```python
from build123d import *

# Parameters (mm, degrees)
SKIZZE1_W                       = 22
SKIZZE1_H                       = 72.8
AUFSATZ_LINEAR_AUSTRAGEN1_DEPTH = 2
SKIZZE2_R                       = 3
SCHNITT_LINEAR_AUSTRAGEN1_DEPTH = 2
SKIZZE3_W                       = 65.5
SKIZZE3_H                       = 21
AUFSATZ_LINEAR_AUSTRAGEN2_DEPTH = 2.8
SCHNITT_LINEAR_AUSTRAGEN2_DEPTH = 67.590464783
SKIZZE5_R                       = 3
SCHNITT_LINEAR_AUSTRAGEN4_DEPTH = 39.128729326
SKIZZE6_W                       = 18
SKIZZE6_H                       = 1
SCHNITT_LINEAR_AUSTRAGEN5_DEPTH = 40
SKIZZE8_W                       = 15
SKIZZE8_H                       = 10
SCHNITT_LINEAR_AUSTRAGEN6_DEPTH = 0.5
VERRUNDUNG3_R                   = 1
SKIZZE9_W                       = 5
SKIZZE9_H                       = 11
AUFSATZ_LINEAR_AUSTRAGEN3_DEPTH = 6
SKIZZE10_W                      = 9
SKIZZE10_H                      = 4
SCHNITT_LINEAR_AUSTRAGEN7_DEPTH = 75.007364498


with BuildPart() as part:
    # Skizze1 → Aufsatz-Linear austragen1 (new body)
    with BuildSketch(Plane(origin=(0, 0, 0), x_dir=(0, 1, 0), z_dir=(0, 0, 1))):
        Rectangle(SKIZZE1_W, SKIZZE1_H)
    extrude(amount=AUFSATZ_LINEAR_AUSTRAGEN1_DEPTH)

    # Skizze2 → Schnitt-Linear austragen1 (cut)
    with BuildSketch(Plane.XY.offset(2)):
        with Locations((-34.28, 8.88)):
            Circle(SKIZZE2_R)
        with Locations((-34.28, -8.88)):
            Circle(SKIZZE2_R)
        with Locations((34.28, -8.88)):
            Circle(SKIZZE2_R)
        with Locations((34.28, 8.88)):
            Circle(SKIZZE2_R)
    extrude(amount=-SCHNITT_LINEAR_AUSTRAGEN1_DEPTH, mode=Mode.SUBTRACT)

    # Skizze3 → Aufsatz-Linear austragen2 (add)
    with BuildSketch(Plane.XY.offset(2)):
        with Locations((3.65, 0)):
            Rectangle(SKIZZE3_W, SKIZZE3_H)
    extrude(amount=AUFSATZ_LINEAR_AUSTRAGEN2_DEPTH)

    # Skizze4 → Schnitt-Linear austragen2 (cut, through all)
    with BuildSketch(Plane(origin=(-29.1, 0, 0), x_dir=(0, -1, 0), z_dir=(-1, 0, 0))):
        Polygon((-8, 4.8), (8, 4.8), (8, 4.1), (9, 4.1), (9, 2), (-9, 2), (-9, 4.1), (-8, 4.1), align=None)
    extrude(amount=-SCHNITT_LINEAR_AUSTRAGEN2_DEPTH, mode=Mode.SUBTRACT)

    # Skizze5 → Schnitt-Linear austragen4 (cut, through all)
    with BuildSketch(Plane(origin=(0, 0, 2), x_dir=(1, 0, 0), z_dir=(0, 0, -1))):
        with Locations((34.28, -8.88)):
            Circle(SKIZZE5_R)
        with Locations((34.28, 8.88)):
            Circle(SKIZZE5_R)
    extrude(amount=-SCHNITT_LINEAR_AUSTRAGEN4_DEPTH, mode=Mode.SUBTRACT)

    # Skizze6 → Schnitt-Linear austragen5 (cut)
    with BuildSketch(Plane(origin=(-36.4, 0, 0), x_dir=(0, -1, 0), z_dir=(-1, 0, 0))):
        with Locations((0, 2)):
            Rectangle(SKIZZE6_W, SKIZZE6_H)
    extrude(amount=-SCHNITT_LINEAR_AUSTRAGEN5_DEPTH, mode=Mode.SUBTRACT)

    # Skizze8 → Schnitt-Linear austragen6 (cut)
    with BuildSketch(Plane.XY.offset(2)):
        with Locations((8.655984658, -0.007335612)):
            Rectangle(SKIZZE8_W, SKIZZE8_H)
    extrude(amount=-SCHNITT_LINEAR_AUSTRAGEN6_DEPTH, mode=Mode.SUBTRACT)

    # Verrundung3
    # the kernel refuses this fillet: 1 mm, written as the material it adds along each edge
    with BuildSketch(Plane(origin=(3.6, -9, 1.5), x_dir=(0, 0, 1), z_dir=(0, 1, 0))) as verrundung3_piece_1:
        with BuildLine():
            CenterArc((1, -0.866025404), VERRUNDUNG3_R, 120, 60)
            Line((0, -0.866025404), (-0.02, -0.866025404))
            Line((-0.02, -0.866025404), (-0.02, 0))
            Line((-0.02, 0), (0, 0.02))
            ThreePointArc((0, 0.02), (0.25, 0.02), (0.49, 0.017320508))
            Line((0.49, 0.017320508), (0.5, 0))
        make_face()
    extrude(amount=3.992664388)
    with BuildSketch(Plane(origin=(3.6, -5.007335612, 1.5), x_dir=(0, 0, 1), z_dir=(1, 0, 0)), Plane(origin=(16.155984658, 4.992664388, 1.5), x_dir=(0, 0, 1), z_dir=(-1, 0, 0))) as verrundung3_piece_2:
        with BuildLine():
            CenterArc((1, -0.866025404), VERRUNDUNG3_R, 120, 60)
            Line((0, -0.866025404), (-0.02, -0.866025404))
            Line((-0.02, -0.866025404), (-0.02, 0))
            Line((-0.02, 0), (0, 0.02))
            ThreePointArc((0, 0.02), (0.25, 0.02), (0.49, 0.017320508))
            Line((0.49, 0.017320508), (0.5, 0))
        make_face()
    extrude(amount=12.555984658)
    with BuildSketch(Plane(origin=(3.6, 4.992664388, 1.5), x_dir=(0, 0, 1), z_dir=(0, 1, 0))) as verrundung3_piece_3:
        with BuildLine():
            CenterArc((1, -0.866025404), VERRUNDUNG3_R, 120, 60)
            Line((0, -0.866025404), (-0.02, -0.866025404))
            Line((-0.02, -0.866025404), (-0.02, 0))
            Line((-0.02, 0), (0, 0.02))
            ThreePointArc((0, 0.02), (0.25, 0.02), (0.49, 0.017320508))
            Line((0.49, 0.017320508), (0.5, 0))
        make_face()
    extrude(amount=4.007335612)
    with BuildSketch(Plane(origin=(16.155984658, -5.007335612, 1.5), x_dir=(0, 0, 1), z_dir=(0, 1, 0))) as verrundung3_piece_4:
        with BuildLine():
            CenterArc((1, -0.866025404), VERRUNDUNG3_R, 120, 60)
            Line((0, -0.866025404), (-0.02, -0.866025404))
            Line((-0.02, -0.866025404), (-0.02, 0))
            Line((-0.02, 0), (0, 0.02))
            ThreePointArc((0, 0.02), (0.25, 0.02), (0.49, 0.017320508))
            Line((0.49, 0.017320508), (0.5, 0))
        make_face()
    extrude(amount=10)
    with BuildSketch(Plane(origin=(3.6, -9, 1.5), x_dir=(0, 0, 1), z_dir=(0, 1, 0))) as verrundung3_piece_5a_section:
        with BuildLine():
            CenterArc((1, -0.866025404), VERRUNDUNG3_R, 120, 60)
            Line((0, -0.866025404), (-0.02, -0.866025404))
            Line((-0.02, -0.866025404), (-0.02, 0))
            Line((-0.02, 0), (0, 0.02))
            ThreePointArc((0, 0.02), (0.25, 0.02), (0.49, 0.017320508))
            Line((0.49, 0.017320508), (0.5, 0))
        make_face()
    verrundung3_piece_5a = extrude(amount=6.157727897, mode=Mode.PRIVATE)
    verrundung3_piece_5a = split(verrundung3_piece_5a, bisect_by=Plane(origin=(3.383689554, -5.007335612, 1.629516711), z_dir=(0, 1, 0)), keep=Keep.TOP, mode=Mode.PRIVATE)
    with BuildSketch(Plane(origin=(1.434936491, -5.007335612, 1.5), x_dir=(0, 0, 1), z_dir=(1, 0, 0))) as verrundung3_piece_5b_section:
        with BuildLine():
            CenterArc((1, -0.866025404), VERRUNDUNG3_R, 120, 60)
            Line((0, -0.866025404), (-0.02, -0.866025404))
            Line((-0.02, -0.866025404), (-0.02, 0))
            Line((-0.02, 0), (0, 0.02))
            ThreePointArc((0, 0.02), (0.25, 0.02), (0.49, 0.017320508))
            Line((0.49, 0.017320508), (0.5, 0))
        make_face()
    verrundung3_piece_5b = extrude(amount=14.721048168, mode=Mode.PRIVATE)
    verrundung3_piece_5b = split(verrundung3_piece_5b, bisect_by=Plane(origin=(3.6, -4.791025166, 1.629516711), z_dir=(-1, 0, 0)), keep=Keep.TOP, mode=Mode.PRIVATE)
    verrundung3_piece_5 = verrundung3_piece_5a & verrundung3_piece_5b
    add(verrundung3_piece_5)
    with BuildSketch(Plane(origin=(3.6, -5.007335612, 1.5), x_dir=(0, 0, 1), z_dir=(1, 0, 0))) as verrundung3_piece_6a_section:
        with BuildLine():
            CenterArc((1, -0.866025404), VERRUNDUNG3_R, 120, 60)
            Line((0, -0.866025404), (-0.02, -0.866025404))
            Line((-0.02, -0.866025404), (-0.02, 0))
            Line((-0.02, 0), (0, 0.02))
            ThreePointArc((0, 0.02), (0.25, 0.02), (0.49, 0.017320508))
            Line((0.49, 0.017320508), (0.5, 0))
        make_face()
    verrundung3_piece_6a = extrude(amount=14.721048168, mode=Mode.PRIVATE)
    verrundung3_piece_6a = split(verrundung3_piece_6a, bisect_by=Plane(origin=(16.155984658, -4.791025166, 1.629516711), z_dir=(1, 0, 0)), keep=Keep.TOP, mode=Mode.PRIVATE)
    with BuildSketch(Plane(origin=(16.155984658, -7.172399122, 1.5), x_dir=(0, 0, 1), z_dir=(0, 1, 0))) as verrundung3_piece_6b_section:
        with BuildLine():
            CenterArc((1, -0.866025404), VERRUNDUNG3_R, 120, 60)
            Line((0, -0.866025404), (-0.02, -0.866025404))
            Line((-0.02, -0.866025404), (-0.02, 0))
            Line((-0.02, 0), (0, 0.02))
            ThreePointArc((0, 0.02), (0.25, 0.02), (0.49, 0.017320508))
            Line((0.49, 0.017320508), (0.5, 0))
        make_face()
    verrundung3_piece_6b = extrude(amount=12.165063509, mode=Mode.PRIVATE)
    verrundung3_piece_6b = split(verrundung3_piece_6b, bisect_by=Plane(origin=(15.939674213, -5.007335612, 1.629516711), z_dir=(0, -1, 0)), keep=Keep.TOP, mode=Mode.PRIVATE)
    verrundung3_piece_6 = verrundung3_piece_6a & verrundung3_piece_6b
    add(verrundung3_piece_6)
    with BuildSketch(Plane(origin=(16.155984658, 4.992664388, 1.5), x_dir=(0, 0, 1), z_dir=(-1, 0, 0))) as verrundung3_piece_7a_section:
        with BuildLine():
            CenterArc((1, -0.866025404), VERRUNDUNG3_R, 120, 60)
            Line((0, -0.866025404), (-0.02, -0.866025404))
            Line((-0.02, -0.866025404), (-0.02, 0))
            Line((-0.02, 0), (0, 0.02))
            ThreePointArc((0, 0.02), (0.25, 0.02), (0.49, 0.017320508))
            Line((0.49, 0.017320508), (0.5, 0))
        make_face()
    verrundung3_piece_7a = extrude(amount=14.721048168, mode=Mode.PRIVATE)
    verrundung3_piece_7a = split(verrundung3_piece_7a, bisect_by=Plane(origin=(3.6, 4.776353942, 1.629516711), z_dir=(-1, 0, 0)), keep=Keep.TOP, mode=Mode.PRIVATE)
    with BuildSketch(Plane(origin=(3.6, 2.827600878, 1.5), x_dir=(0, 0, 1), z_dir=(0, 1, 0))) as verrundung3_piece_7b_section:
        with BuildLine():
            CenterArc((1, -0.866025404), VERRUNDUNG3_R, 120, 60)
            Line((0, -0.866025404), (-0.02, -0.866025404))
            Line((-0.02, -0.866025404), (-0.02, 0))
            Line((-0.02, 0), (0, 0.02))
            ThreePointArc((0, 0.02), (0.25, 0.02), (0.49, 0.017320508))
            Line((0.49, 0.017320508), (0.5, 0))
        make_face()
    verrundung3_piece_7b = extrude(amount=6.172399122, mode=Mode.PRIVATE)
    verrundung3_piece_7b = split(verrundung3_piece_7b, bisect_by=Plane(origin=(3.383689554, 4.992664388, 1.629516711), z_dir=(0, -1, 0)), keep=Keep.TOP, mode=Mode.PRIVATE)
    verrundung3_piece_7 = verrundung3_piece_7a & verrundung3_piece_7b
    add(verrundung3_piece_7)
    with BuildSketch(Plane(origin=(16.155984658, -5.007335612, 1.5), x_dir=(0, 0, 1), z_dir=(0, 1, 0))) as verrundung3_piece_8a_section:
        with BuildLine():
            CenterArc((1, -0.866025404), VERRUNDUNG3_R, 120, 60)
            Line((0, -0.866025404), (-0.02, -0.866025404))
            Line((-0.02, -0.866025404), (-0.02, 0))
            Line((-0.02, 0), (0, 0.02))
            ThreePointArc((0, 0.02), (0.25, 0.02), (0.49, 0.017320508))
            Line((0.49, 0.017320508), (0.5, 0))
        make_face()
    verrundung3_piece_8a = extrude(amount=12.165063509, mode=Mode.PRIVATE)
    verrundung3_piece_8a = split(verrundung3_piece_8a, bisect_by=Plane(origin=(15.939674213, 4.992664388, 1.629516711), z_dir=(0, 1, 0)), keep=Keep.TOP, mode=Mode.PRIVATE)
    with BuildSketch(Plane(origin=(18.321048168, 4.992664388, 1.5), x_dir=(0, 0, 1), z_dir=(-1, 0, 0))) as verrundung3_piece_8b_section:
        with BuildLine():
            CenterArc((1, -0.866025404), VERRUNDUNG3_R, 120, 60)
            Line((0, -0.866025404), (-0.02, -0.866025404))
            Line((-0.02, -0.866025404), (-0.02, 0))
            Line((-0.02, 0), (0, 0.02))
            ThreePointArc((0, 0.02), (0.25, 0.02), (0.49, 0.017320508))
            Line((0.49, 0.017320508), (0.5, 0))
        make_face()
    verrundung3_piece_8b = extrude(amount=14.721048168, mode=Mode.PRIVATE)
    verrundung3_piece_8b = split(verrundung3_piece_8b, bisect_by=Plane(origin=(16.155984658, 4.776353942, 1.629516711), z_dir=(1, 0, 0)), keep=Keep.TOP, mode=Mode.PRIVATE)
    verrundung3_piece_8 = verrundung3_piece_8a & verrundung3_piece_8b
    add(verrundung3_piece_8)

    # Skizze9 → Aufsatz-Linear austragen3 (add)
    with BuildSketch(Plane.XY.offset(1.5)):
        with Locations((-33.9, 0)):
            Rectangle(SKIZZE9_W, SKIZZE9_H)
    extrude(amount=AUFSATZ_LINEAR_AUSTRAGEN3_DEPTH)

    # Skizze10 → Schnitt-Linear austragen7 (cut, through all)
    with BuildSketch(Plane(origin=(-36.4, 0, 0), x_dir=(0, -1, 0), z_dir=(-1, 0, 0))):
        with Locations((0.038201858, 5)):
            Rectangle(SKIZZE10_W, SKIZZE10_H)
    extrude(amount=-SCHNITT_LINEAR_AUSTRAGEN7_DEPTH, mode=Mode.SUBTRACT)


solid = part.part
```
Source: CAD feature listing. Evaluate the final solid. Frame: model axes, mm. A direction names the side the tool comes from. Coordinates: 2 decimals unless noted, no trailing zeros. Loops run counter-clockwise (first coordinate to the right, second up) from the corner with the lowest first, then second, coordinate; pieces in that order, holes last. Notation, with made-up numbers: M 61.5,30 L 103.5,30 A25 ccw 103.5,46 Z; hole C 36,5 d11. An arc over 180 degrees is marked long. Put each result on its own line as item: value. Start each with the question number.
1) Cut plane B-B on x = -11.5. Return the cut outline in (y, z), then the cut area to 3 significant figures.
2) Reachability of faces 4 (the face through (-29.1, 10, 4)), 5 (the face through (-31.4, 0, 2)), 6 (the face through (0, 9, 3)), 7 (the face through (-34, 0, 7)), 8 (the face through (1, 10.5, 3)) from +Z, -Z, +X, -X, +Y, -Y: full face, straight path, thin tool, end or side. Return the list, or none.
3) Contact query for flat-ended pins moving along their axis: pin 1 Ø0.8 at (x, z) = (10.5, 3.5) entering from +Y; pin 2 Ø1 at (x, y) = (-1.5, -4) entering from +Z; pin 3 Ø1.4 at (x, z) = (8.5, 3) entering from -Y; pin 4 Ø12 at (x, y) = (9, -7) entering from -Z. Output: stop coordinate, or through.
4) Cut plane D-D on x = 34.28. Return the cut outline in (y, z), then the cut area to 3 significant figures.
5) Cut plane C-C on x = 13.5. Return the cut outline in (y, z).
6) Ray query, L1, parallel to Y at x = -2, z = 3.25; L2, parallel to Z at x = -27.5, y = -1.75; L3, parallel to Y at x = -2.5, z = 4.25. Return the intervals inside material, ascending. Write a range as from..to.
7) Cut plane A-A on x = -34.28. Return the cut outline in (y, z), then the cut area to 3 significant figures.
8) Pull-direction query (Y, two-part tool) for faces 1 (the face through (-34, 4.462, 5)), 2 (the face through (1, -10.5, 3)), 3 (the face through (1, -9, 4.8)); classes: pulls with the +Y half, pulls with the -Y half, needs draft (parallel to the pull), parting line crosses it, or undercut.
The answers:
1. outline: M -11,0 L 11,0 L 11,2 L 10.5,2 L 10.5,4.8 L 8,4.8 L 8,4.1 L 9,4.1 L 9,1.5 L -9,1.5 L -9,4.1 L -8,4.1 L -8,4.8 L -10.5,4.8 L -10.5,2 L -11,2 Z
1. area: 44.8 mm²
2. face 4: +Z, -X, +Y, -Y
2. face 5: +Z
2. face 6: -X
2. face 7: +X, -X
2. face 8: +Z, +X, -X, +Y
3. pin 1: stops at y = 10.5
3. pin 2: stops at z = 1.5
3. pin 3: stops at y = -10.5
3. pin 4: stops at z = 0
4. outline: M -5.88,0 L 5.88,0 L 5.88,2 L -5.88,2 Z
4. area: 23.5 mm²
5. outline: M -11,0 L 11,0 L 11,2 L 10.5,2 L 10.5,4.8 L 8,4.8 L 8,4.1 L 9,4.1 L 9,2 L 4.99,2 A1 cw 4.13,1.5 L -4.14,1.5 A1 cw -5.01,2 L -9,2 L -9,4.1 L -8,4.1 L -8,4.8 L -10.5,4.8 L -10.5,2 L -11,2 Z
6. L1: y = -10.5..-9, 9..10.5
6. L2: z = 0..1.5
6. L3: y = -10.5..-8, 8..10.5
7. outline: M -5.88,0 L 5.88,0 L 5.88,1.5 L 5.5,1.5 L 5.5,7.5 L -5.5,7.5 L -5.5,1.5 L -5.88,1.5 Z; hole M -4.54,3 L 4.46,3 L 4.46,7 L -4.54,7 Z
7. area: 47.6 mm²
8. face 1: undercut
8. face 2: pulls with the -Y half
8. face 3: needs draft
